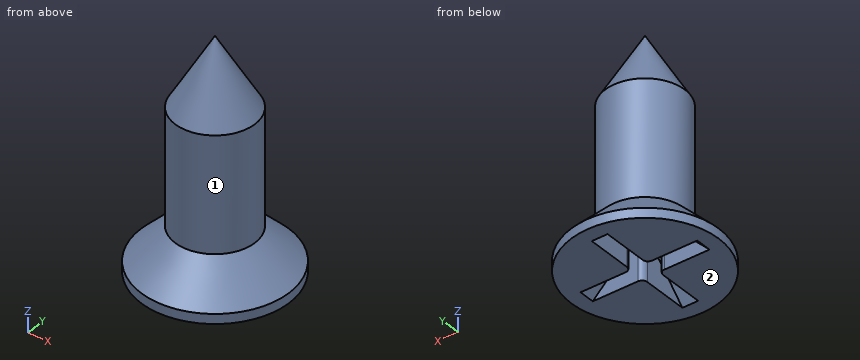
from build123d import *

# Parameters (mm, degrees)
CUT_EXTRUDE1_DEPTH = 1.737
DRAFT1_ANGLE       = 45


with BuildPart() as part:
    # Sketch1 → Revolve1 (revolve)
    with BuildSketch(Plane(origin=(0, 0, 0), x_dir=(1, 0, 0), z_dir=(0, 1, 0))):
        Polygon((0, 0), (0, -10), (0.01, -10), (1.75, -6.986231595), (1.75, -1.93), (3.25, -0.43), (3.25, 0), align=None)
    revolve(axis=Axis((0, 0, 0), (0, 0, -1)))

    # Sketch2 → Cut-Extrude1 (cut)
    with BuildSketch(Plane(origin=(0, 0, 0), x_dir=(-1, 0, 0), z_dir=(0, 0, -1))):
        with BuildLine():
            Line((-0.35, 0.583333333), (-0.35, 0.845898975))
            Line((-0.35, 0.845898975), (0.35, 0.845898975))
            Line((0.35, 0.845898975), (0.35, 0.583333333))
            ThreePointArc((0.35, 0.583333333), (0.418341751, 0.418341751), (0.583333333, 0.35))
            Line((0.583333333, 0.35), (0.845898975, 0.35))
            Line((0.845898975, 0.35), (0.845898975, -0.35))
            Line((0.845898975, -0.35), (0.583333333, -0.35))
            ThreePointArc((0.583333333, -0.35), (0.418341751, -0.418341751), (0.35, -0.583333333))
            Line((0.35, -0.583333333), (0.35, -0.845898975))
            Line((0.35, -0.845898975), (-0.35, -0.845898975))
            Line((-0.35, -0.845898975), (-0.35, -0.583333333))
            ThreePointArc((-0.35, -0.583333333), (-0.418341751, -0.418341751), (-0.583333333, -0.35))
            Line((-0.583333333, -0.35), (-0.845898975, -0.35))
            Line((-0.845898975, -0.35), (-0.845898975, 0.35))
            Line((-0.845898975, 0.35), (-0.583333333, 0.35))
            ThreePointArc((-0.583333333, 0.35), (-0.418341751, 0.418341751), (-0.35, 0.583333333))
        make_face()
    extrude(amount=-CUT_EXTRUDE1_DEPTH, mode=Mode.SUBTRACT)

    # Draft1
    draft1_faces = [part.faces().sort_by_distance(p)[0] for p in [
        (0, -0.845898975, 0.8685),
        (-0.845898975, 0, 0.8685),
        (0.845898975, 0, 0.8685),
        (0, 0.845898975, 0.8685),
    ]]
    draft(draft1_faces, Plane(origin=(-0.583333333, 0.583333333, 1.737), x_dir=(-1, 0, 0), z_dir=(0, 0, -1)), DRAFT1_ANGLE)


solid = part.part
Can you work these out from the model? Positions are in its coordinate system, mm. Face numbers are marked on the shaded views. A direction names the side the tool comes from. Give positions to 0.01 mm unless a question says otherwise; leave off trailing zeros. Loops run counter-clockwise (first coordinate to the right, second up) from the corner with the lowest first, then second, coordinate; pieces in that order, holes last. Notation, with made-up numbers: (9.5, 88) - (64.5, 88) arc R16 ccw to (64.5, 104) - close; hole circle Ø11 at (-33, 76). An arc over 180 degrees is marked (long way). Return JSON: item names as keys, results as strings.
1. I want a section at A-A on z = 2.5. Please give me the cut outline in (x, y), and give its area (3 significant figures).
Output values:
{"outline": "circle Ø3.5 at (0, 0)", "area": "9.62 mm²"}
2. If I drill on line 1 (X direction, y = 0.5, z = 1); line 2 (X direction, y = 0, z = 2.5); line 3 (Y direction, x = -0.25, z = 3.25), over which ranges is the centre line in solid material (lowest first)?
Output values:
{"line 1": "x = -2.63 to -0.37, 0.37 to 2.63", "line 2": "x = -1.75 to 1.75", "line 3": "y = -1.73 to 1.73"}
3. I want a section at B-B on z = 8.5. Please give me the cut outline in (x, y).
Output values:
{"outline": "circle Ø1.75 at (0, 0)"}
4. I'm going to push flat-ended pins straight in: pin 1 Ø3 at (y, z) = (-1.5, 5) entering from +X; pin 2 Ø0.5 at (y, z) = (2, 0.5) entering from +X; pin 3 Ø1.9 at (x, z) = (1.5, 1) entering from +Y. Where does each tip first touch, or does it pass through?
Output values:
{"pin 1": "stops at x = 1.75", "pin 2": "stops at x = 2.73", "pin 3": "stops at y = 3.16"}
5. For the marked faces 1 and 2, which set-ups out of +Z, -Z, +X, -X, +Y, -Y let a thin tool reach every point of the face, with its end or its side?
Output values:
{"face 1": "+Z", "face 2": "-Z, +X, -X, +Y, -Y"}
